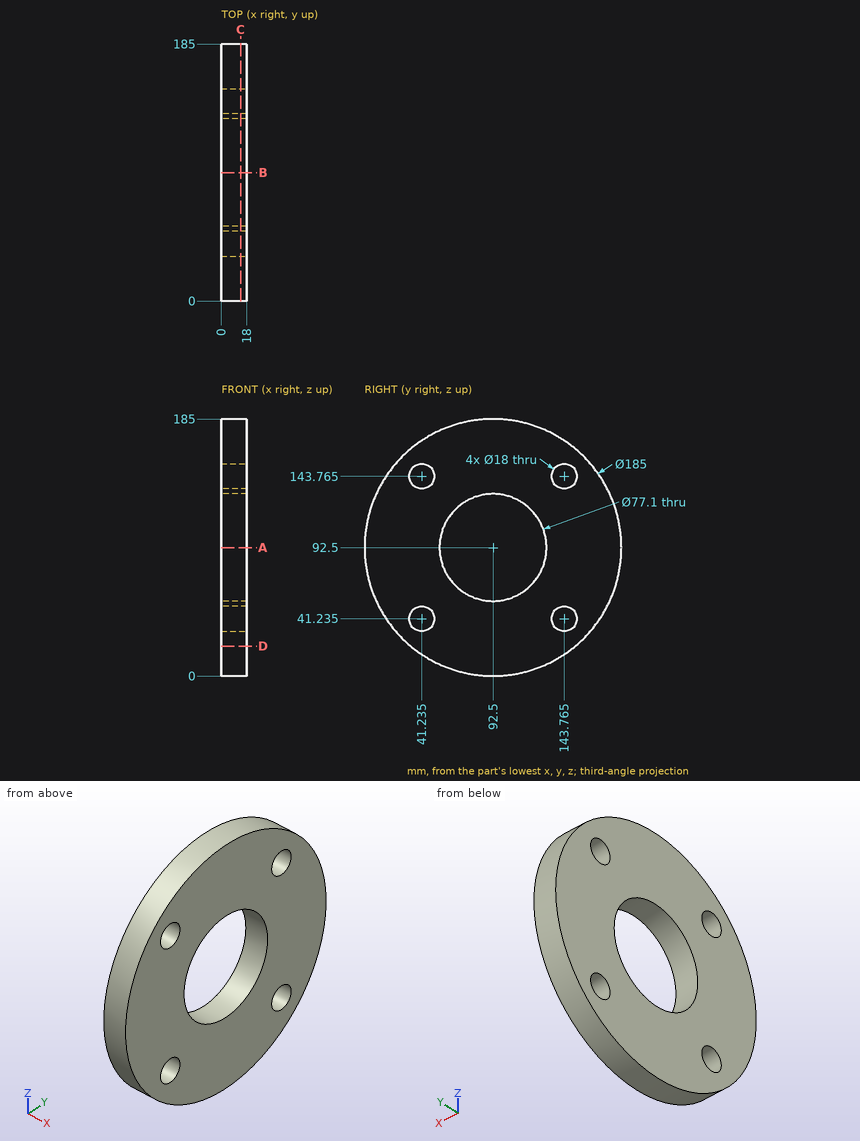
Can you work these out from the drawing? Everything is in mm from the part's minimum corner. Coordinates: 2 decimals unless noted, no trailing zeros. Order: outer loops, then holes, each group sorted by start corner. A loop starts at its lowest first (then second) coordinate and runs counter-clockwise, first axis right, second up. Notation, with made-up numbers: (32.5, -10.75) -> (45.5, -10.75) arc R18 cw to (45.5, 2.25) -> close; hole circle Ø2 at (79, 13.25). An arc over 180 degrees is marked (long way). Return JSON: item names as keys, results as strings.
1) If I drill on probe 1 along Z at (x, y) = (11, 38.5); probe 2 along Y at (x, z) = (16.5, 46); probe 3 along Z at (x, y) = (7.75, 144.5) (1 decimal), over which ranges is the centre line in solid material (lowest first)?
Conclusion:
{"probe 1": "z = 17.4 to 32.66, 49.81 to 135.19, 152.34 to 167.6", "probe 2": "y = 12.54 to 33.6, 48.87 to 136.13, 151.4 to 172.46", "probe 3": "z = 16 to 32.3, 50.2 to 134.8, 152.7 to 169"}
2) If we section it at A-A on z = 92.5: List the corners of the cut face in (x, y) for me.
Conclusion:
{"outline": "(0, 0) -> (18, 0) -> (18, 53.95) -> (0, 53.95) -> close; (0, 131.05) -> (18, 131.05) -> (18, 185) -> (0, 185) -> close"}
3) If we section it at C-C on x = 13.75: State how many separate pieces and enclosed holes the cut face has, plus the area to 3 significant figures.
Conclusion:
{"separate pieces": "1", "enclosed holes": "5", "area": "21,200 mm²"}
4) I'm going to push flat-ended pins straight in: P1, Ø2, axis at x = 4, z = 103, coming from the +Y side; P2, Ø1, axis at y = 161.5, z = 32, coming from the -X side; P3, Ø2, axis at x = 5.5, y = 52.5, coming from the -Z side; P4, Ø8, axis at x = 16, y = 84, coming from the -Z side. Where does each tip first touch, or does it pass through?
Conclusion:
{"P1": "stops at y = 184.51", "P2": "stops at x = 0", "P3": "stops at z = 8.62", "P4": "stops at z = 0.11"}
5) If we section it at D-D on z = 21.5: List the corners of the cut face in (x, y) for me, plus the area to 3 significant figures.
Conclusion:
{"outline": "(0, 33.21) -> (18, 33.21) -> (18, 151.79) -> (0, 151.79) -> close", "area": "2,130 mm²"}
